from build123d import *

# Parameters (mm, degrees)
SKETCH_1_W                  = 5
SKETCH_1_H                  = 11.6
EXTRUDE_1_DEPTH             = 30
SKETCH_2_W                  = 5
SKETCH_2_H                  = 11.6
EXTRUDE_2_DEPTH             = 6
HOLE_WIZARD_M3_1_D          = 2.5
HOLE_WIZARD_M3_1_DEPTH      = 7.5
HOLE_WIZARD_M3_1_TIP        = 0.751075774
HOLE_WIZARD_1_D             = 2.4
HOLE_WIZARD_1_DEPTH         = 7.5
HOLE_WIZARD_1_CBORE_D       = 4.3
HOLE_WIZARD_1_CBORE_DEPTH   = 2.3
HOLE_WIZARD_1_TIP           = 0.721032743
FILLET_1_R                  = 0.5
HOLE_WIZARD_3_2_3_2_1_D     = 3.2
HOLE_WIZARD_3_2_3_2_1_DEPTH = 5.2
HOLE_WIZARD_3_2_3_2_1_TIP   = 0.96137699
HOLE_WIZARD_M2_1_D          = 1.6
HOLE_WIZARD_M2_1_DEPTH      = 5.2
HOLE_WIZARD_M2_1_TIP        = 0.480688495


with BuildPart() as part:
    # 草图1 → 凸台-拉伸1 (new body, symmetric)
    with BuildSketch(Plane.XY):
        Rectangle(SKETCH_1_W, SKETCH_1_H)
    extrude(amount=EXTRUDE_1_DEPTH, both=True)

    # 草图2 → 凸台-拉伸2 (add)
    with BuildSketch(Plane(origin=(2.5, 0, 0), x_dir=(0, 0, -1), z_dir=(1, 0, 0))):
        with Locations((-27.5, 0)):
            Rectangle(SKETCH_2_W, SKETCH_2_H)
    extrude_2 = extrude(amount=EXTRUDE_2_DEPTH)

    # 镜向1: 凸台-拉伸2 across plane
    add(extrude_2.mirror(Plane.XY))

    # M3 螺纹孔1
    with Locations(Plane.XY.offset(30)):
        with Locations((4.5, -3), (4.5, 3)):
            Hole(HOLE_WIZARD_M3_1_D / 2, depth=HOLE_WIZARD_M3_1_DEPTH)
            with Locations((0, 0, -(HOLE_WIZARD_M3_1_DEPTH + HOLE_WIZARD_M3_1_TIP / 2))):  # 118° drill point
                Cone(0, HOLE_WIZARD_M3_1_D / 2, HOLE_WIZARD_M3_1_TIP, mode=Mode.SUBTRACT)

    # 打孔尺寸(%根据)内六角圆柱头螺钉的类型1
    with Locations(Plane.XY.offset(-25)):
        with Locations((5.5, -3), (5.5, 3)):
            CounterBoreHole(HOLE_WIZARD_1_D / 2, HOLE_WIZARD_1_CBORE_D / 2, HOLE_WIZARD_1_CBORE_DEPTH, depth=HOLE_WIZARD_1_DEPTH)
            with Locations((0, 0, -(HOLE_WIZARD_1_DEPTH + HOLE_WIZARD_1_TIP / 2))):  # 118° drill point
                Cone(0, HOLE_WIZARD_1_D / 2, HOLE_WIZARD_1_TIP, mode=Mode.SUBTRACT)

    # 圆角1
    fillet_1_edges = [part.edges().sort_by_distance(p)[0] for p in [
        (2.5, 0, 25),
        (2.5, 0, -25),
        (-2.5, 0, 30),
        (-2.5, 0, -30),
    ]]
    fillet(fillet_1_edges, radius=FILLET_1_R)

    # Ø3.2 (3.2) 直径孔1
    with Locations(Plane.ZY.offset(2.5)):
        with Locations((1.6, 0.8)):
            Hole(HOLE_WIZARD_3_2_3_2_1_D / 2, depth=HOLE_WIZARD_3_2_3_2_1_DEPTH)
            with Locations((0, 0, -(HOLE_WIZARD_3_2_3_2_1_DEPTH + HOLE_WIZARD_3_2_3_2_1_TIP / 2))):  # 118° drill point
                Cone(0, HOLE_WIZARD_3_2_3_2_1_D / 2, HOLE_WIZARD_3_2_3_2_1_TIP, mode=Mode.SUBTRACT)

    # M2 螺纹孔1
    with Locations(Plane(origin=(0, -5.8, 0), x_dir=(-1, 0, 0), z_dir=(0, -1, 0))):
        with Locations((-0.325, 9)):
            Hole(HOLE_WIZARD_M2_1_D / 2, depth=HOLE_WIZARD_M2_1_DEPTH)
            with Locations((0, 0, -(HOLE_WIZARD_M2_1_DEPTH + HOLE_WIZARD_M2_1_TIP / 2))):  # 118° drill point
                Cone(0, HOLE_WIZARD_M2_1_D / 2, HOLE_WIZARD_M2_1_TIP, mode=Mode.SUBTRACT)


solid = part.part
Check sheet for the modelled part. Datum: model origin and axes. Units: mm. A direction names the side the tool comes from. Round coordinates to 2 decimals unless told otherwise and drop trailing zeros. Loops run counter-clockwise (first coordinate to the right, second up) from the corner with the lowest first, then second, coordinate; pieces in that order, holes last. Notation, with made-up numbers: (50.25, 60.5) -> (105.25, 60.5) arc R21 ccw to (105.25, 97.5) -> close; hole circle Ø6 at (-28.75, 67.25). An arc over 180 degrees is marked (long way). Put each result on its own line as item: value. Start each with the question number.
1. Gauge pin test, flat ends, axial feed: pin 1 (2.5 mm diameter, centred on x = 0.325, z = -9, fed in from -Y); pin 2 (3 mm diameter, centred on y = 0.8, z = 1.6, fed in from +X). Record the tip position at first contact, or that the pin passes through.
2. Access from +Z, -Z, +X, -X, +Y, -Y to the whole of each face (thin tool, end or side, straight path). Record for faces 4 (the face through (5.421, 3.845, 27.465)), 5 (the face through (5.5, 1.6, -27.3)), 6 (the face through (6.7, -2.95, -28.67)), 7 (the face through (6, 0, -25)), 8 (the face through (0, -5.8, 0)).
3. Section check A-A (y = -3). Enter the section's corners in (x, z) (3 decimals).
4. Section check D-D (z = 9.5). Enter the section's corners in (x, y).
5. Section check C-C (z = 1.5). Enter the section's corners in (x, y).
6. Scan lines: probe 1 along Y at (x, z) = (4.5, 26); probe 2 along Y at (x, z) = (5.5, -26.65); probe 3 along X at (y, z) = (-4.1, -9) (3 decimals). Record each from-to range of solid material in increasing order.
7. Section check B-B (y = 3). Enter the section's corners in (x, z), plus the area to 3 significant figures.
8. Draft check along Z on faces 1 (the face through (0.221, -3.164, -9.793)), 2 (the face through (3, 0, -30)), 3 (the face through (0, 5.8, 0)). Enter one of: +Z half, -Z half, draft (parallel to the pull), parting line (faces both ways), or undercut.
Findings:
1. pin 1: stops at y = -5.8
1. pin 2: passes through
2. face 4: +Z
2. face 5: none
2. face 6: -Z
2. face 7: +X, +Y, -Y
2. face 8: +Z, -Z, +X, -X, -Y
3. outline: (-2.5, -29.5) arc R0.5 ccw to (-2, -30) -> (4.3, -30) -> (4.3, -27.3) -> (3.35, -27.3) -> (3.35, -25) -> (3, -25) arc R0.5 cw to (2.5, -24.5) -> (2.5, 24.5) arc R0.5 cw to (3, 25) -> (3.25, 25) -> (3.25, 30) -> (-2, 30) arc R0.5 ccw to (-2.5, 29.5) -> close; (5.75, 25) -> (8.5, 25) -> (8.5, 30) -> (5.75, 30) -> close; (6.7, -30) -> (8.5, -30) -> (8.5, -25) -> (7.65, -25) -> (7.65, -27.3) -> (6.7, -27.3) -> close; hole circle Ø1.6 at (0.325, -9)
4. outline: (-2.5, -5.8) -> (2.5, -5.8) -> (2.5, 5.8) -> (-2.5, 5.8) -> close
5. outline: (-2.5, -5.8) -> (2.5, -5.8) -> (2.5, -0.8) -> (-2.5, -0.8) -> close; (-2.5, 2.4) -> (2.5, 2.4) -> (2.5, 5.8) -> (-2.5, 5.8) -> close
6. probe 1: y = -5.8 to -4.25, -1.75 to 1.75, 4.25 to 5.8
6. probe 2: y = -5.8 to -5.15, -0.85 to 0.85, 5.15 to 5.8
6. probe 3: x = -2.5 to -0.475, 1.125 to 2.5
7. outline: (-2.5, -29.5) arc R0.5 ccw to (-2, -30) -> (4.3, -30) -> (4.3, -27.3) -> (3.35, -27.3) -> (3.35, -25) -> (3, -25) arc R0.5 cw to (2.5, -24.5) -> (2.5, 24.5) arc R0.5 cw to (3, 25) -> (3.25, 25) -> (3.25, 30) -> (-2, 30) arc R0.5 ccw to (-2.5, 29.5) -> close; (5.75, 25) -> (8.5, 25) -> (8.5, 30) -> (5.75, 30) -> close; (6.7, -30) -> (8.5, -30) -> (8.5, -25) -> (7.65, -25) -> (7.65, -27.3) -> (6.7, -27.3) -> close
7. area: 331 mm^2
8. face 1: undercut
8. face 2: -Z half
8. face 3: draft
